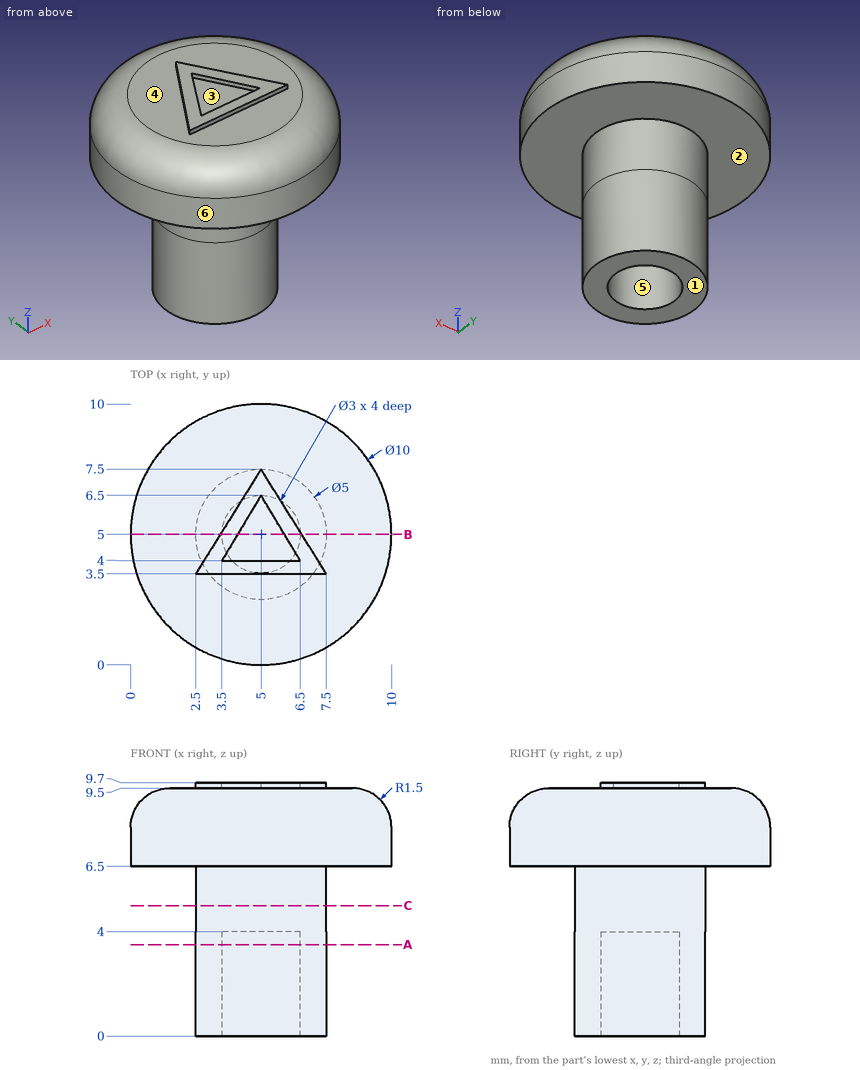
Geometry: see drawing. Coordinates: mm, zero at the bounding-box minimum. A direction names the side the tool comes from. Round coordinates to 2 decimals unless told otherwise and drop trailing zeros. Write each loop counter-clockwise with the first axis right and the second up, starting at its lowest first coordinate (ties: lowest second). Pieces come first, ordered by that corner, then holes.
Item 1: Mould query, pull axis X, two halves, no side actions, for the marked faces 3, 4, 5 and 6. Classes: +X half, -X half, draft (parallel to the pull), parting line (faces both ways), or undercut.
Item 2: Pin query (flat end, axial travel): P1, Ø0.9, axis at x = 4.5, y = 5, coming from the -Z side; P2, Ø1.5, axis at x = 7, y = 1.5, coming from the +Z side; P3, Ø1.5, axis at y = 6.5, z = 7.5, coming from the +X side. Return the tip coordinate at first contact, or that it passes through.
Item 3: Section query B-B (y = 5). Return loops of the section in (x, z).
Item 4: Section query A-A (z = 3.5). Return loops of the section in (x, y), plus the area to 3 significant figures.
Item 5: Set-up query: the marked faces 1 and 2. Return all of +Z, -Z, +X, -X, +Y, -Y with unobstructed straight access to the full face (end or side cutting, diameter ignored); none if empty.
Item 6: Material intervals for L1, parallel to Y at x = 5, z = 2.5; L2, parallel to Z at x = 6.25, y = 7.25, sorted ascending.
Item 7: Section query C-C (z = 5). Return loops of the section in (x, y), plus the area to 3 significant figures.
Completed:
1. face 3: undercut
1. face 4: draft
1. face 5: undercut
1. face 6: parting line
2. P1: stops at z = 4
2. P2: stops at z = 9.5
2. P3: stops at x = 9.94
3. outline: (0, 6.5) - (2.5, 6.5) - (2.5, 0) - (3.5, 0) - (3.5, 4) - (6.5, 4) - (6.5, 0) - (7.5, 0) - (7.5, 6.5) - (10, 6.5) - (10, 8) arc R1.5 ccw to (8.5, 9.5) - (6.56, 9.5) - (6.56, 9.7) - (5.9, 9.7) - (5.9, 9.5) - (4.1, 9.5) - (4.1, 9.7) - (3.44, 9.7) - (3.44, 9.5) - (1.5, 9.5) arc R1.5 ccw to (0, 8) - close
4. outline: circle Ø5 at (5, 5); hole circle Ø3 at (5, 5)
4. area: 12.6 mm2
5. face 1: -Z, +X, -X, +Y, -Y
5. face 2: -Z
6. L1: y = 2.5 to 3.5, 6.5 to 7.5
6. L2: z = 6.5 to 9.5
7. outline: circle Ø5 at (5, 5)
7. area: 19.6 mm2
